from build123d import *

# Parameters (mm, degrees)
SKETCH_1_R          = 40
SKETCH_1_R_2        = 1.25
EXTRUDE_1_DEPTH     = 10
SKETCH_2_R          = 2.4
CUT_EXTRUDE_1_DEPTH = 6
CUT_EXTRUDE_2_DEPTH = 58.445626465


with BuildPart() as part:
    # 草图1 → 凸台-拉伸1 (new body)
    with BuildSketch(Plane(origin=(0, 0, 0), x_dir=(1, 0, 0), z_dir=(0, 1, 0))):
        with Locations(Location((0, 0, 0), (0, 0, 270))):
            Circle(SKETCH_1_R)
        with Locations(Location((6.75, 0, 0), (0, 0, 270))):
            Circle(SKETCH_1_R_2, mode=Mode.SUBTRACT)
        with Locations(Location((0, -6.75, 0), (0, 0, 270))):
            Circle(SKETCH_1_R_2, mode=Mode.SUBTRACT)
        with Locations(Location((-6.75, 0, 0), (0, 0, 270))):
            Circle(SKETCH_1_R_2, mode=Mode.SUBTRACT)
        with Locations(Location((0, 6.75, 0), (0, 0, 270))):
            Circle(SKETCH_1_R_2, mode=Mode.SUBTRACT)
    extrude(amount=EXTRUDE_1_DEPTH)

    # 草图2 → 切除-拉伸1 (cut)
    with BuildSketch(Plane(origin=(0, 10, 0), x_dir=(1, 0, 0), z_dir=(0, 1, 0))):
        with Locations(Location((0, 6.75, 0), (0, 0, 270))):
            Circle(SKETCH_2_R)
        with Locations(Location((6.75, 0, 0), (0, 0, 270))):
            Circle(SKETCH_2_R)
        with Locations(Location((0, -6.75, 0), (0, 0, 270))):
            Circle(SKETCH_2_R)
        with Locations(Location((-6.75, 0, 0), (0, 0, 270))):
            Circle(SKETCH_2_R)
    extrude(amount=-CUT_EXTRUDE_1_DEPTH, mode=Mode.SUBTRACT)

    # 草图3 → 切除-拉伸2 (cut, through all)
    with BuildSketch(Plane(origin=(0, 10, 0), x_dir=(1, 0, 0), z_dir=(0, 1, 0))):
        with BuildLine():
            Line((20, 0), (35, 0))
            ThreePointArc((35, 0), (24.748737342, -24.748737342), (0, -35))
            Line((0, -35), (0, -20))
            ThreePointArc((0, -20), (14.142135624, -14.142135624), (20, 0))
        make_face()
    extrude(amount=-CUT_EXTRUDE_2_DEPTH, mode=Mode.SUBTRACT)


solid = part.part
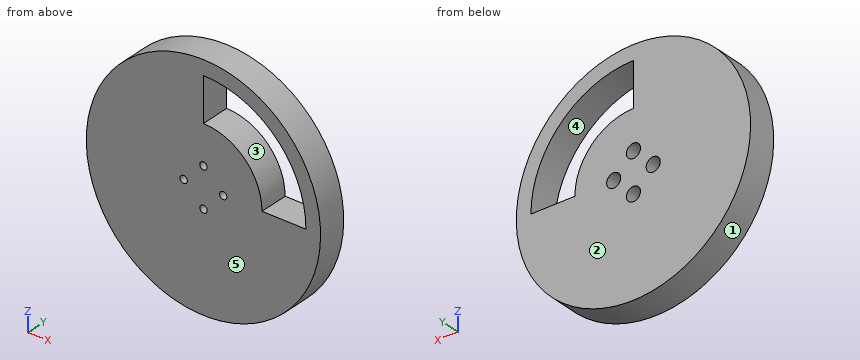
Design review of the part built by this model. Coordinates are the model's own, in mm. Face numbers are marked on the shaded views. A direction names the side the tool comes from. Give positions to 0.01 mm unless a question says otherwise; leave off trailing zeros. Write each loop counter-clockwise with the first axis right and the second up, starting at its lowest first coordinate (ties: lowest second). Pieces come first, ordered by that corner, then holes. Notation, with made-up numbers: M 16.5,35 L 21.5,35 A23 cw 21.5,45 Z; hole C 60,57 d10. An arc over 180 degrees is marked long. Answer as a JSON object with one key per item and string values. Group by question number.
1) We need section C-C (x = -6.75). Give the boundary of the cut face in (y, z).
2) We need section A-A (y = 2). Give the boundary of the cut face in (x, z).
3) Clearance check with flat-ended pins moving along their axes: pin 1 Ø3 at (x, y) = (-15.5, 4) entering from -Z; pin 2 Ø2 at (x, z) = (0, 6.75) entering from -Y; pin 3 Ø2.5 at (x, z) = (0, 6.5) entering from +Y; pin 4 Ø1.5 at (x, y) = (-17.5, 5.5) entering from -Z. State where each tip first meets the part, or that it passes through.
4) We need section B-B (z = -6.75). Give the boundary of the cut face in (x, y), and give its area (3 significant figures).
5) For line 1 along X through (y, z) = (7.25, 7) (3 decimals); line 2 along X through (y, z) = (5, -1.5); line 3 along X through (y, z) = (0.75, 12.5), list the stretches that pass through material, from the lowest coordinate up.
6) Tool access review of the marked faces 4 and 5: name each direction out of +Z, -Z, +X, -X, +Y, -Y from which nothing blocks a thin tool from reaching the whole face with its end or side.
7) Mouldability with a two-part tool opening along X and no side actions: class the marked faces 1, 2 and 3 as released by +X, released by -X, zero draft, split by the parting line, or undercut.
8) We need section D-D (z = 6.75). Give the boundary of the cut face in (x, y).
Answer key:
{
 "1": {"outline": "M 0,-39.43 L 10,-39.43 L 10,-2.4 L 4,-2.4 L 4,-1.25 L 0,-1.25 Z; M 0,1.25 L 4,1.25 L 4,2.4 L 10,2.4 L 10,39.43 L 0,39.43 Z"},
 "2": {"outline": "C 0,0 d80; hole C -6.75,0 d2.5; hole C 0,-6.75 d2.5; hole C 0,6.75 d2.5; hole M 0,20 A20 cw 20,0 L 35,0 A35 ccw 0,35 Z; hole C 6.75,0 d2.5"},
 "3": {"pin 1": "stops at z = -37.47", "pin 2": "passes through", "pin 3": "stops at y = 4", "pin 4": "stops at z = -36.32"},
 "4": {"outline": "M -39.43,0 L -1.25,0 L -1.25,4 L -2.4,4 L -2.4,10 L -39.43,10 Z; M 1.25,0 L 39.43,0 L 39.43,10 L 2.4,10 L 2.4,4 L 1.25,4 Z", "area": "750 mm²"},
 "5": {"line 1": "x = -39.383 to -2.387, 2.387 to 18.735, 34.293 to 39.383", "line 2": "x = -39.97 to -8.62, -4.88 to 4.88, 8.62 to 39.97", "line 3": "x = -38 to 15.61, 32.69 to 38"},
 "6": {"face 4": "+Y, -Y", "face 5": "+Z, -Z, +X, -X, -Y"},
 "7": {"face 1": "split by the parting line", "face 2": "zero draft", "face 3": "undercut"},
 "8": {"outline": "M -39.43,0 L -1.25,0 L -1.25,4 L -2.4,4 L -2.4,10 L -39.43,10 Z; M 1.25,0 L 18.83,0 L 18.83,10 L 2.4,10 L 2.4,4 L 1.25,4 Z; M 34.34,0 L 39.43,0 L 39.43,10 L 34.34,10 Z"}
}
